```python
from build123d import *

# Parameters (mm, degrees)
F1_DEPTH = 6.35
F2_R     = 6.35
F3_DEPTH = 53.975
F4_R     = 1.27


with BuildPart() as f1:
    # F0 (on Front) → F1 (new body)
    with BuildSketch(Plane.XZ):
        Polygon((-5.499261, 9.525), (-10.998523, 0), (-5.499261, -9.525), (5.499261, -9.525), (10.998523, 0), (5.499261, 9.525), align=None)
    extrude(amount=F1_DEPTH)

    # F2 (on face) → F3 (join)
    with BuildSketch(Plane(origin=(0, 0, 0), x_dir=(-1, 0, 0), z_dir=(0, 1, 0))):
        Circle(F2_R)
    extrude(amount=F3_DEPTH)

    # F4
    f4_edges = [f1.edges().sort_by_distance(p)[0] for p in [
        (6.35, 53.975, 0),
    ]]
    fillet(f4_edges, radius=F4_R)


solid = f1.part
```
Part model, mm, in its own coordinate system. A direction names the side the tool comes from. Round coordinates to 2 decimals unless told otherwise and drop trailing zeros. Write each loop counter-clockwise with the first axis right and the second up, starting at its lowest first coordinate (ties: lowest second). Pieces come first, ordered by that corner, then holes. Notation, with made-up numbers: M 56.5,2.5 L 97.5,2.5 A20 ccw 97.5,27.5 Z; hole C 1.25,68.25 d6. An arc over 180 degrees is marked long. Answer as CSV lines item,"result". Start each with the question number.
1) Drop flat-ended pins along their axis: pin 1 (1.5 mm diameter, centred on x = 4, y = 27.5, fed in from -Z); pin 2 (1.5 mm diameter, centred on x = -3.5, y = 6, fed in from +Z); pin 3 (6 mm diameter, centred on x = 5.5, y = 20, fed in from +Z). Give the stop position or say it passes through.
2) Band-saw the part on B-B (y = 39). List the corners of the cut face in (x, z), then the cut area to 3 significant figures.
3) Drill centre lines: L1, parallel to X at y = 28, z = -0.25; L2, parallel to Y at x = -2.25, z = 8.75. Where is each one in solid material? Low to high.
4) Which spindle directions (+Z, -Z, +X, -X, +Y, -Y) get a long thin tool onto all of the face, cutting with end or side? Do faces 1 (the face through (0, 53.975, 0)), 2 (the face through (-0.2, 0, 6.5)). Say none if no direction does.
5) Band-saw the part on A-A (x = 0). List the corners of the cut face in (y, z) (3 decimals).
6) Band-saw the part on C-C (x = -7.25). List the corners of the cut face in (y, z).
Worked out:
1,pin 1,"z = -5.46"
1,pin 2,"z = 5.72"
1,pin 3,"z = 5.84"
2,outline,"C 0,0 d12.7"
2,area,"127 mm²"
3,L1,"-6.35 to 6.35"
3,L2,"-6.35 to 0"
4,face 1,"+Z, -Z, +X, -X, +Y"
4,face 2,"+Y"
5,outline,"M -6.35,-9.525 L 0,-9.525 L 0,-6.35 L 52.705,-6.35 A1.27 ccw 53.975,-5.08 L 53.975,5.08 A1.27 ccw 52.705,6.35 L 0,6.35 L 0,9.525 L -6.35,9.525 Z"
6,outline,"M -6.35,-6.49 L 0,-6.49 L 0,6.49 L -6.35,6.49 Z"
